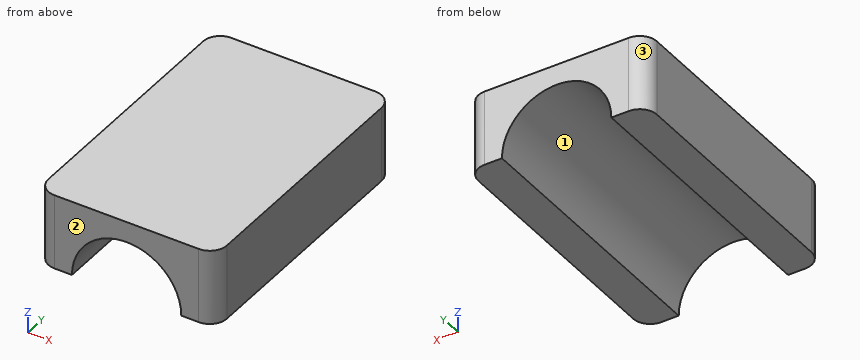
```python
from build123d import *

# Parameters (mm, degrees)
ESQUISSE1_W             = 52.2
ESQUISSE1_H             = 80
BOSS_EXTRU_2_DEPTH      = 22
CONG_2_R                = 5
ESQUISSE2_R             = 16
ENL_V_MAT_EXTRU_3_DEPTH = 93.647092521


with BuildPart() as part:
    # Esquisse1 → Boss.-Extru.2 (new body)
    with BuildSketch(Plane.XY):
        with Locations((-15.124795362, -42.006460905)):
            Rectangle(ESQUISSE1_W, ESQUISSE1_H)
    extrude(amount=BOSS_EXTRU_2_DEPTH)

    # Congé2
    cong_2_edges = [part.edges().sort_by_distance(p)[0] for p in [
        (-41.224795362, -2.006460905, 11),
        (10.975204638, -2.006460905, 11),
        (10.975204638, -82.006460905, 11),
        (-41.224795362, -82.006460905, 11),
    ]]
    fillet(cong_2_edges, radius=CONG_2_R)

    # Esquisse2 → Enlèv. mat.-Extru.3 (cut, through all)
    with BuildSketch(Plane.XZ.offset(82.006460905)):
        with Locations((-15.124795362, 0)):
            Circle(ESQUISSE2_R)
    extrude(amount=-ENL_V_MAT_EXTRU_3_DEPTH, mode=Mode.SUBTRACT)


solid = part.part
```
Source: CAD feature listing. Evaluate the final solid. Frame: model axes, mm. Face numbers are marked on the shaded views. Coordinates: 2 decimals unless noted, no trailing zeros. Write each loop counter-clockwise with the first axis right and the second up, starting at its lowest first coordinate (ties: lowest second). Pieces come first, ordered by that corner, then holes. Notation, with made-up numbers: (30, 1.5) - (39, 1.5) arc R31 cw to (39, 31.5) - close; hole circle Ø6 at (34.5, 65). An arc over 180 degrees is marked (long way). Answer as a JSON object with one key per item and string values.
Q1. Section query D-D, the plane x = -25. Output: boundary loops of the cut face in (y, z).
Ans:
{"outline": "(-82.01, 12.59) - (-2.01, 12.59) - (-2.01, 22) - (-82.01, 22) - close"}
Q2. Section query C-C, the plane z = 8. Output: boundary loops of the cut face in (x, y), plus the area to 3 significant figures.
Ans:
{"outline": "(-41.22, -77.01) arc R5 ccw to (-36.22, -82.01) - (-28.98, -82.01) - (-28.98, -2.01) - (-36.22, -2.01) arc R5 ccw to (-41.22, -7.01) - close; (-1.27, -82.01) - (5.98, -82.01) arc R5 ccw to (10.98, -77.01) - (10.98, -7.01) arc R5 ccw to (5.98, -2.01) - (-1.27, -2.01) - close", "area": "1,940 mm2"}
Q3. First-contact query: pin 1 Ø6 at (x, y) = (-2, -17) entering from -Z; pin 2 Ø4 at (x, z) = (-3, 2.5) entering from -Y. Flat tips, straight axial feed; report the tip coordinate or a pass-through.
Ans:
{"pin 1": "stops at z = 0", "pin 2": "passes through"}
Q4. Section query B-B, the plane y = -21. Output: boundary loops of the cut face in (x, z).
Ans:
{"outline": "(-41.22, 0) - (-31.12, 0) arc R16 cw to (0.88, 0) - (10.98, 0) - (10.98, 22) - (-41.22, 22) - close"}
Q5. Draft query along X for the marked faces 1, 2 and 3. Return one class per face: released by +X, released by -X, zero draft, split by the parting line, or undercut.
Ans:
{"face 1": "undercut", "face 2": "zero draft", "face 3": "released by -X"}
Q6. Material intervals for line 1 (X direction, y = -10, z = 10.5); line 2 (X direction, y = -72, z = 6.5); line 3 (Z direction, x = -11.5, y = -16.5), sorted ascending. Write a range as [from, to].
Ans:
{"line 1": "x = [-41.22, -27.2], [-3.05, 10.98]", "line 2": "x = [-41.22, -29.74], [-0.5, 10.98]", "line 3": "z = [15.58, 22]"}
Q7. Section query A-A, the plane z = 12. Output: boundary loops of the cut face in (x, y), plus the area to 3 significant figures.
Ans:
{"outline": "(-41.22, -77.01) arc R5 ccw to (-36.22, -82.01) - (-25.71, -82.01) - (-25.71, -2.01) - (-36.22, -2.01) arc R5 ccw to (-41.22, -7.01) - close; (-4.54, -82.01) - (5.98, -82.01) arc R5 ccw to (10.98, -77.01) - (10.98, -7.01) arc R5 ccw to (5.98, -2.01) - (-4.54, -2.01) - close", "area": "2,460 mm2"}
